Read the model definition and answer for the solid it produces. Units are mm, in the model's axes. A direction names the side the tool comes from. Give positions to 0.01 mm unless a question says otherwise; leave off trailing zeros. Order: outer loops, then holes, each group sorted by start corner. A loop starts at its lowest first (then second) coordinate and runs counter-clockwise, first axis right, second up.
Item 1: Find the intervals of material crossed by line 1 along Y through (x, z) = (0, 47); line 2 along X through (y, z) = (-29, 28.5); line 3 along Z through (x, y) = (8, -51.5), in increasing order.
Item 2: A cutting plane is placed at D-D (x = -30). Write down the section's boundary in (y, z).
Item 3: A cutting plane is placed at A-A (x = 36). Write down the section's boundary in (y, z), plus the area to 3 significant figures.
Item 4: A cutting plane is placed at B-B (y = 3). Write down the section's boundary in (x, z).
Item 5: Which of the six approach directions +Z, -Z, +X, -X, +Y, -Y give full straight-line access (tool end or side, diameter ignored) to faces 1 (the face through (0, 4, 75)), 2 (the face through (71.994, -3, 28)), 3 (the face through (71.12, -3.1, 75.6)), 4 (the face through (-36.314, 38.731, 65.737))?
Item 6: A cutting plane is placed at C-C (z = 9). Write down the section's boundary in (x, y).
Item 7: Given pin 1 Ø1 at (y, z) = (46.5, 24) entering from -X; pin 2 Ø3 at (x, z) = (-48.5, 38.5) entering from +Y; pin 3 Ø1 at (x, y) = (-15.5, -49.5) entering from +Z, each flat-ended and moving along its own axis, determine where each tip first touches the part or whether it passes through.
from build123d import *

# Parameters (mm, degrees)
F0_W      = 144.5718035102
F0_H      = 98.2272140682
F1_DEPTH  = 63.5
F3_DEPTH  = 73.66
F1_FACE_W = 98.2272140682
F1_FACE_H = 55.8175444603
F5_DEPTH  = 73.66
F7_DEPTH  = 71.12
F9_DEPTH  = 73.66


with BuildPart() as f1:
    # F0 (on Top) → F1 (new body)
    with BuildSketch(Plane.XY):
        with Locations((-0.2914778888, -2.040328458)):
            Rectangle(F0_W, F0_H)
    extrude(amount=F1_DEPTH)

    # F2 (on Right) → F3 (join)
    with BuildSketch(Plane.YZ):
        Polygon((-77.5057077408, 55.8175444603), (76.3933062553, 55.8175444603), (0, 76.2208253145), align=None)
    extrude(amount=F3_DEPTH)

    # F4 (on Right) + F3_face (on face) + F1_face (on face) → F5 (join)
    with BuildSketch(Plane.YZ):
        Polygon((0, 75.6378695369), (-76.9227594137, 56.1090186238), (76.3933062553, 56.1090186238), align=None)
    with BuildSketch(Plane(origin=(73.66, -0.3708004951, 62.6186380784), x_dir=(0, 1, 0), z_dir=(1, 0, 0))):
        Polygon((-77.1349072456, -6.8010936181), (76.7641067505, -6.8010936181), (0.3708004951, 13.6021872362), align=None)
    with BuildSketch(Plane(origin=(71.9944238663, -2.040328458, 27.9087722301), x_dir=(0, 1, 0), z_dir=(1, 0, 0))):
        Rectangle(F1_FACE_W, F1_FACE_H)
    extrude(amount=-F5_DEPTH)

    # F6 (on Right) → F7 (join)
    with BuildSketch(Plane.YZ):
        Polygon((-76.9643932581, 55.8175444603), (76.6431465745, 55.8175444603), (0, 76.8037736416), align=None)
    extrude(amount=F7_DEPTH)

    # F8 (on Right) + F5_face (on face) → F9 (join)
    with BuildSketch(Plane.YZ):
        Polygon((0, 76.2208253145), (-76.6312852502, 56.1090186238), (76.6847804189, 56.1090186238), align=None)
    with BuildSketch(Plane(origin=(-73.66, -0.1764843861, 62.6186355948), x_dir=(0, 1, 0), z_dir=(-1, 0, 0))):
        Polygon((-76.7462750276, 6.509616971), (0.1764843861, -13.019233942), (76.5697906415, 6.509616971), align=None)
    extrude(amount=F9_DEPTH, dir=(1, 0, 0))


solid = f1.part
Response values:
1. line 1: y = -51.15 to 47.07
1. line 2: x = -72.58 to 71.99
1. line 3: z = 55.82 to 62.76
2. outline: (-76.92, 56.11) - (-51.15, 56.11) - (-51.15, 0) - (47.07, 0) - (47.07, 56.11) - (76.39, 56.11) - (0, 75.64) - (-47.81, 63.5) - (-51.15, 63.5) - (-51.15, 62.65) - close
3. outline: (-77.51, 55.82) - (-51.15, 55.82) - (-51.15, 0) - (47.07, 0) - (47.07, 55.82) - (76.64, 55.82) - (75.58, 56.11) - (76.68, 56.11) - (50.47, 62.99) - (0, 76.8) - (-48.79, 63.5) - (-51.15, 63.5) - (-51.15, 62.86) - (-57.01, 61.26) - (-76.63, 56.11) - (-76.4, 56.11) - close
3. area: 7,100 mm2
4. outline: (-73.66, 56.11) - (-72.58, 56.11) - (-72.58, 0) - (71.99, 0) - (71.99, 55.82) - (73.66, 55.82) - (73.66, 75.43) - (71.12, 75.43) - (71.12, 75.98) - (0, 75.98) - (0, 74.87) - (-73.66, 74.87) - close
5. face 1: +Z, -X
5. face 2: -Z, +X, +Y, -Y
5. face 3: +Z, +X
5. face 4: +Z, -X, +Y
6. outline: (-72.58, -51.15) - (71.99, -51.15) - (71.99, 47.07) - (-72.58, 47.07) - close
7. pin 1: stops at x = -72.58
7. pin 2: stops at y = 47.07
7. pin 3: stops at z = 63.5
